CAD build for the part. Positions are in the model's coordinates, mm. A direction names the side the tool comes from. Give positions to 0.01 mm unless a question says otherwise; leave off trailing zeros. Loops run counter-clockwise (first coordinate to the right, second up) from the corner with the lowest first, then second, coordinate; pieces in that order, holes last.
Item 1: Probe probe 1 along Y at (x, z) = (13.3, 2.15); probe 2 along X at (y, z) = (97, 2.7); probe 3 along X at (y, z) = (14.5, 8.5). List the from-to ranges inside material, lowest first.
Item 2: Saw through at C-C on z = 3. Give the number of separate pieces and of enclosed holes in the cut face, plus the area to 3 significant figures.
Item 3: Which spindle directions (+Z, -Z, +X, -X, +Y, -Y) get a long thin tool onto all of the face, cutting with end or side? Do faces 4 (the flat face through (15, 23, 12.1)), 5 (the flat face through (18, 23, 7)), 6 (the flat face through (0, 2, 2)). Say none if no direction does.
Item 4: Saw through at A-A on y = 81.5. Give the cut face in (x, z), plus the area to 3 significant figures.
Item 5: Saw through at D-D on y = 7. Give the cut face in (x, z), plus the area to 3 significant figures.
Item 6: Drop flat-ended pins along their axis: P1, Ø7, axis at y = 23.5, z = 11, coming from the -X side; P2, Ø1, axis at y = 58, z = 2.5, coming from the +X side; P3, Ø8, axis at x = 0, y = -2, coming from the +Z side. Give the stop position or say it passes through.
Item 7: Mould opens along Z. For faces 1 (the flat face through (0, 52, 2)), 2 (the flat face through (15, 24, 14)), 3 (the flat face through (14, 23, 10)) say: released by +Z, released by -Z, zero draft, split by the parting line, or undercut.
Item 8: Saw through at B-B on x = -13. Give the cut face in (y, z), plus the area to 3 significant figures.
from build123d import *

# Parameters (mm, degrees)
SKETCH1_R               = 2.55
BOSS_EXTRUDE1_DEPTH     = 5
SKETCH2_W               = 6
SKETCH2_H               = 46.7
BOSS_EXTRUDE2_DEPTH     = 9
BOSS_EXTRUDE3_DEPTH     = 3
SKETCH4_R               = 1.75
CUT_EXTRUDE1_DEPTH      = 65.060049953
CUT_EXTRUDE2_DEPTH      = 68.578768855
CUT_EXTRUDE2_DEPTH_BACK = 68.578768855
SKETCH6_W               = 43
SKETCH6_H               = 43
BOSS_EXTRUDE4_DEPTH     = 5
SKETCH8_R               = 1.5
SKETCH8_R_2             = 12
CUT_EXTRUDE3_DEPTH      = 115.841847773
BOSS_EXTRUDE5_START     = -5
BOSS_EXTRUDE5_DEPTH     = 5


with BuildPart() as part:
    # Sketch1 → Boss-Extrude1 (new body)
    with BuildSketch(Plane.XY):
        with BuildLine():
            Line((0, 0), (34, 0))
            Line((34, 0), (34, 3))
            ThreePointArc((34, 3), (32, 7), (34, 11))
            Line((34, 11), (34, 42.7))
            ThreePointArc((34, 42.7), (32, 46.7), (34, 50.7))
            Line((34, 50.7), (34, 53.7))
            Line((34, 53.7), (0, 53.7))
            Line((0, 53.7), (0, 50.7))
            ThreePointArc((0, 50.7), (2, 46.7), (0, 42.7))
            Line((0, 42.7), (0, 11))
            ThreePointArc((0, 11), (2, 7), (0, 3))
            Line((0, 3), (0, 0))
        make_face()
        with Locations((7, 46.7)):
            Circle(SKETCH1_R, mode=Mode.SUBTRACT)
        with Locations((27, 46.7)):
            Circle(SKETCH1_R, mode=Mode.SUBTRACT)
        with Locations((7, 7)):
            Circle(SKETCH1_R, mode=Mode.SUBTRACT)
        with Locations((27, 7)):
            Circle(SKETCH1_R, mode=Mode.SUBTRACT)
    extrude(amount=BOSS_EXTRUDE1_DEPTH)

    # Sketch2 → Boss-Extrude2 (add)
    with BuildSketch(Plane.XY.offset(5)):
        with Locations((15, 23.35)):
            Rectangle(SKETCH2_W, SKETCH2_H)
    extrude(amount=BOSS_EXTRUDE2_DEPTH)

    # Sketch3 → Boss-Extrude3 (add)
    with BuildSketch(Plane.XY.offset(5)):
        with BuildLine():
            Line((12, -10), (12, 5.8))
            Line((12, 5.8), (11.85386444, 5.8))
            ThreePointArc((11.85386444, 5.8), (7, 2), (2.14613556, 5.8))
            Line((2.14613556, 5.8), (-15.8, 5.8))
            Line((-15.8, 5.8), (-15.8, -10))
            Line((-15.8, -10), (12, -10))
        make_face()
    extrude(amount=BOSS_EXTRUDE3_DEPTH)

    # Sketch4 → Cut-Extrude1 (cut, through all)
    with BuildSketch(Plane.XY.offset(8)):
        with Locations((9.2, 3)):
            Circle(SKETCH4_R)
        with Locations((-13, -7.2)):
            Circle(SKETCH4_R)
    extrude(amount=-CUT_EXTRUDE1_DEPTH, mode=Mode.SUBTRACT)

    # Sketch5 → Cut-Extrude2 (cut, two sides: drawn at the far end of the back side and taken through both)
    with BuildSketch(Plane(origin=(0, 46.7, 0), x_dir=(1, 0, 0), z_dir=(0, 1, 0)).offset(-CUT_EXTRUDE2_DEPTH_BACK)):
        Polygon((98.816452891, -8.55), (18, -8.55), (16.1, -8.55), (16.1, -7), (14, -7), (14, -12.1), (16.1, -12.1), (16.1, -10.55), (18, -10.55), (98.816452891, -10.55), (260.449358672, -10.55), (260.449358672, -8.55), align=None)
    extrude(amount=CUT_EXTRUDE2_DEPTH + CUT_EXTRUDE2_DEPTH_BACK, mode=Mode.SUBTRACT)

    # Sketch6 → Boss-Extrude4 (add, through all)
    with BuildSketch(Plane.XY.offset(5)):
        with Locations((29.1, 81.2)):
            Rectangle(SKETCH6_W, SKETCH6_H)
        Polygon((34, 53.7), (50.6, 59.7), (7.6, 59.7), (0, 53.7), align=None)
    extrude(amount=-BOSS_EXTRUDE4_DEPTH)

    # Sketch8 → Cut-Extrude3 (cut, through all)
    with BuildSketch(Plane.XY.offset(5)):
        with Locations((13.3, 97)):
            Circle(SKETCH8_R)
        with Locations((44.3, 97)):
            Circle(SKETCH8_R)
        with Locations((13.3, 66)):
            Circle(SKETCH8_R)
        with Locations((44.3, 66)):
            Circle(SKETCH8_R)
        with Locations((28.8, 81.5)):
            Circle(SKETCH8_R_2)
    extrude(amount=-CUT_EXTRUDE3_DEPTH, mode=Mode.SUBTRACT)

    # Sketch9 → Boss-Extrude5 (add)
    with BuildSketch(Plane.XY.offset(5).offset(BOSS_EXTRUDE5_START)):
        with BuildLine():
            Line((34, 11), (50.6, 59.7))
            Line((50.6, 59.7), (34, 53.7))
            Line((34, 53.7), (34, 50.7))
            ThreePointArc((34, 50.7), (39.236067977, 51.172135955), (42, 46.7))
            ThreePointArc((42, 46.7), (39.236067977, 42.227864045), (34, 42.7))
            Line((34, 42.7), (34, 11))
        make_face()
    extrude(amount=BOSS_EXTRUDE5_DEPTH)


solid = part.part
Results below:
1. probe 1: y = 0 to 64.5, 67.5 to 95.5, 98.5 to 102.7
1. probe 2: x = 7.6 to 11.8, 14.8 to 42.8, 45.8 to 50.6
1. probe 3: x = 12 to 14, 16.1 to 18
2. separate pieces: 1
2. enclosed holes: 11
2. area: 3,580 mm2
3. face 4: +Y, -Y
3. face 5: +Z, +X, +Y, -Y
3. face 6: -Z, -X, +Y, -Y
4. outline: (7.6, 0) - (16.8, 0) - (16.8, 5) - (7.6, 5) - close; (40.8, 0) - (50.6, 0) - (50.6, 5) - (40.8, 5) - close
4. area: 95.0 mm2
5. outline: (2, 0) - (4.45, 0) - (4.45, 5) - (2, 5) - close; (9.55, 0) - (24.45, 0) - (24.45, 5) - (18, 5) - (18, 8.55) - (16.1, 8.55) - (16.1, 7) - (14, 7) - (14, 12.1) - (16.1, 12.1) - (16.1, 10.55) - (18, 10.55) - (18, 14) - (12, 14) - (12, 5) - (9.55, 5) - close; (29.55, 0) - (32, 0) - (32, 5) - (29.55, 5) - close
5. area: 138 mm2
6. P1: stops at x = 12
6. P2: stops at x = 50.19
6. P3: stops at z = 8
7. face 1: zero draft
7. face 2: released by +Z
7. face 3: undercut
8. outline: (-10, 5) - (-8.95, 5) - (-8.95, 8) - (-10, 8) - close; (-5.45, 5) - (5.8, 5) - (5.8, 8) - (-5.45, 8) - close
8. area: 36.9 mm2
